Part model, mm, in its own coordinate system. Face numbers are marked on the shaded views. A direction names the side the tool comes from. Coordinates: 2 decimals unless noted, no trailing zeros. Write each loop counter-clockwise with the first axis right and the second up, starting at its lowest first coordinate (ties: lowest second). Pieces come first, ordered by that corner, then holes. Notation, with made-up numbers: (10, 23.5) -> (16, 23.5) arc R13 ccw to (16, 37.5) -> close; hole circle Ø9 at (-28.75, -21.5). An arc over 180 degrees is marked (long way). Write item = value, one per line. Start each with the question number.
Q1. Probe line 1 (Z direction, x = -141.25, y = -28.75); line 2 (X direction, y = -26, z = -141); line 3 (X direction, y = -30, z = 82.5). List the from-to ranges inside material, lowest first.
Q2. Pull direction Z, two halves, no side cores. Call the marked faces 1, 2 and 3: released by +Z, released by -Z, zero draft, split by the parting line, or undercut.
Q3. Band-saw the part on B-B, the plane z = -141.25. List the corners of the cut face in (x, y), plus the area to 3 significant figures.
Q4. Band-saw the part on D-D, the plane y = -32. Give the number of separate pieces and of enclosed holes in the cut face, plus the area to 3 significant figures.
Q5. Pin check, flat tips, straight feed: P1, Ø15.5, axis at x = 15, z = -141.25, coming from the +Y side; P2, Ø6, axis at x = -88.5, y = 18.5, coming from the -Z side; P3, Ø12, axis at x = -33, y = -27, coming from the +Z side. Stop position of each tip, or through.
Q6. Tool access for the marked faces 4, 5, 6, 7 and 8: list every direction of +Z, -Z, +X, -X, +Y, -Y with a clear straight run to the whole face (end or side of a thin tool).
Q7. Band-saw the part on C-C, the plane x = 15. List the corners of the cut face in (y, z).
Q8. Band-saw the part on A-A, the plane x = 141.25. List the corners of the cut face in (y, z).
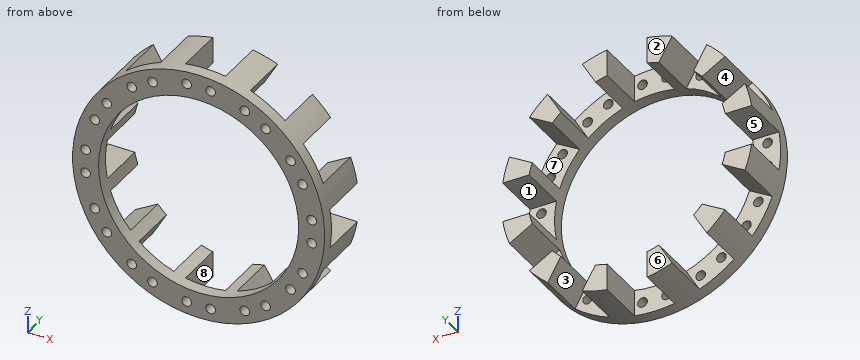
from build123d import *

# Parameters (mm, degrees)
SKETCH1_R           = 157.5
SKETCH1_R_2         = 125
BOSS_EXTRUDE1_DEPTH = 37.5
SKETCH2_W           = 50
SKETCH2_H           = 60
CUT_EXTRUDE1_DEPTH  = 226.873305196
CIRPATTERN1_COUNT   = 12
SKETCH3_R           = 6
CUT_EXTRUDE2_DEPTH  = 236.02659424
CIRPATTERN2_COUNT   = 12


with BuildPart() as part:
    # Sketch1 → Boss-Extrude1 (new, symmetric)
    with BuildSketch(Plane(origin=(0, 0, 0), x_dir=(1, 0, 0), z_dir=(0, 1, 0))):
        with Locations(Location((0, 0, 0), (0, 0, 270))):
            Circle(SKETCH1_R)
        with Locations(Location((0, 0, 0), (0, 0, 270))):
            Circle(SKETCH1_R_2, mode=Mode.SUBTRACT)
    extrude(amount=BOSS_EXTRUDE1_DEPTH, both=True)

    # Sketch2 → Cut-Extrude1 (cut, symmetric)
    with BuildSketch(Plane.XY):
        with Locations((0, 7.5)):
            Rectangle(SKETCH2_W, SKETCH2_H)
    cut_extrude1 = extrude(amount=CUT_EXTRUDE1_DEPTH, both=True, mode=Mode.SUBTRACT)

    # CirPattern1: Cut-Extrude1 ×12 about axis
    cirpattern1_axis = Axis((0, 0, 0), (0, 1, 0))
    for i in range(1, CIRPATTERN1_COUNT):
        add(cut_extrude1.rotate(cirpattern1_axis, i * 360 / CIRPATTERN1_COUNT), mode=Mode.SUBTRACT)

    # Sketch3 → Cut-Extrude2 (cut, through all)
    with BuildSketch(Plane.XZ.offset(37.5)):
        with Locations(Location((-15, 141.25, 0), (0, 0, 270))):
            Circle(SKETCH3_R)
        with Locations(Location((15, 141.25, 0), (0, 0, 270))):
            Circle(SKETCH3_R)
    cut_extrude2 = extrude(amount=-CUT_EXTRUDE2_DEPTH, mode=Mode.SUBTRACT)

    # CirPattern2: Cut-Extrude2 ×12 about axis
    cirpattern2_axis = Axis((0, 0, 0), (0, 1, 0))
    for i in range(1, CIRPATTERN2_COUNT):
        add(cut_extrude2.rotate(cirpattern2_axis, i * 360 / CIRPATTERN2_COUNT), mode=Mode.SUBTRACT)


solid = part.part
Ans:
q1.line_1 = -69.68 to -21, -9 to 9, 21 to 69.68
q1.line_2 = -70.18 to -20.99, -9.01 to 9.01, 20.99 to 70.18
q1.line_3 = -134.16 to -120.72, -108.93 to -93.91, 93.91 to 108.93, 120.72 to 134.16
q2.face_1 = undercut
q2.face_2 = zero draft
q2.face_3 = released by -Z
q3.outline = (-69.68, -37.5) -> (-21, -37.5) -> (-21, -22.5) -> (-25, -22.5) -> (-25, 37.5) -> (-52.68, 37.5) -> (-52.68, -22.5) -> (-69.68, -22.5) -> close; (-9, -37.5) -> (9, -37.5) -> (9, -22.5) -> (-9, -22.5) -> close; (21, -37.5) -> (69.68, -37.5) -> (69.68, -22.5) -> (52.68, -22.5) -> (52.68, 37.5) -> (25, 37.5) -> (25, -22.5) -> (21, -22.5) -> close
q3.area = 5,050 mm2
q4.separate_pieces = 1
q4.enclosed_holes = 25
q4.area = 26,100 mm2
q5.P1 = -22.5
q5.P2 = -108.48
q5.P3 = 155.17
q6.face_4 = -X, +Y
q6.face_5 = +X, -X, +Y
q6.face_6 = +Z, -Z, +X, -X, +Y
q6.face_7 = +Y
q6.face_8 = +Z, -Z, +Y
q7.outline = (-37.5, -156.78) -> (-22.5, -156.78) -> (-22.5, -147.25) -> (-37.5, -147.25) -> close; (-37.5, -135.25) -> (-22.5, -135.25) -> (-22.5, -124.1) -> (-37.5, -124.1) -> close; (-37.5, 124.1) -> (-22.5, 124.1) -> (-22.5, 135.25) -> (-37.5, 135.25) -> close; (-37.5, 147.25) -> (-22.5, 147.25) -> (-22.5, 156.78) -> (-37.5, 156.78) -> close
q8.outline = (-37.5, -69.68) -> (-22.5, -69.68) -> (-22.5, -52.68) -> (37.5, -52.68) -> (37.5, -25) -> (-22.5, -25) -> (-22.5, -21) -> (-37.5, -21) -> close; (-37.5, -9) -> (-22.5, -9) -> (-22.5, 9) -> (-37.5, 9) -> close; (-37.5, 21) -> (-22.5, 21) -> (-22.5, 25) -> (37.5, 25) -> (37.5, 52.68) -> (-22.5, 52.68) -> (-22.5, 69.68) -> (-37.5, 69.68) -> close
